Can you work these out from the model? Positions are in its coordinate system, mm. Round coordinates to 2 decimals unless told otherwise and drop trailing zeros. Order: outer loops, then holes, each group sorted by start corner. A loop starts at its lowest first (then second) coordinate and runs counter-clockwise, first axis right, second up. Notation, with made-up numbers: M 4.25,52.5 L 41.25,52.5 A22 ccw 41.25,87.5 Z; hole C 18.25,65 d4. An arc over 180 degrees is marked long. One line per question, with ' | ' between items.
```python
from build123d import *

# Parameters (mm, degrees)
F1_DEPTH = 260


with BuildPart() as f1:
    # F0 (on Front) → F1 (new body)
    with BuildSketch(Plane.XZ):
        Polygon((0, 20), (0, 0), (100, 0), (100, 10), (100, 20), align=None)
        Polygon((100, 20), (100, 10), (150, 10), align=None)
        Polygon((100, 10), (100, 0), (150, 10), align=None)
    extrude(amount=F1_DEPTH)


solid = f1.part
```
(1) Please list where these lines run through material, in increasing order: probe 1 along Z at (x, y) = (115.5, -44.5); probe 2 along Z at (x, y) = (115, -235). Write a range as [from, to].
Final values:
probe 1: [3.1, 16.9] | probe 2: [3, 17]
(2) If we section it at A-A on y = -145: Please give me the cut outline in (x, z).
Final values:
outline: M 0,0 L 100,0 L 150,10 L 100,20 L 0,20 Z
(3) If we section it at C-C on x = 126: Please give me the cut outline in (y, z), plus the area to 3 significant figures.
Final values:
outline: M -260,5.2 L 0,5.2 L 0,14.8 L -260,14.8 Z | area: 2,500 mm^2
(4) Will these pins go through, and if not, where does the flat tip stop? pin 1 Ø8 at (x, y) = (132.5, -85.5) entering from +Z; pin 2 Ø12 at (x, y) = (109.5, -51) entering from +Z.
Final values:
pin 1: z = 14.3 | pin 2: z = 19.3
(5) If we section it at B-B on z = 2.5: Please give me the cut outline in (x, y), plus the area to 4 significant figures.
Final values:
outline: M 0,-260 L 112.5,-260 L 112.5,0 L 0,0 Z | area: 29,250 mm^2
